Autodesk Inventor part; units mm, degrees
ref_plane "YZ Plane" through (0, 0, 0) normal (1, 0, 0) x (0, 1, 0)
ref_plane "XZ Plane" through (0, 0, 0) normal (0, 1, 0) x (-1, 0, 0)
ref_plane "XY Plane" through (0, 0, 0) normal (0, 0, 1) x (1, 0, 0)
sketch "Skizze1" plane through (0, 0, 0) normal (0, 1, 0) x (-1, 0, 0)
  line L0 (0, 0) -> (216, 0)
  line L1 (216, 0) -> (216, -42.3)
  line L2 (216, -42.3) -> (0, -42.3)
  line L3 (0, -42.3) -> (0, 0)
  dimension "d0" = 216
  dimension "d1" = 42.3
extrude "Extrusion1" add sketch "Skizze1" along normal blind 3
sketch "Skizze2" plane through (0, 6, 3) normal (0, 0, 1) x (1, 0, 0)
  line L0 (-216, 0) -> (0, 0)
  line L1 (0, 0) -> (0, 14)
  line L2 (0, 14) -> (-216, 14)
  line L3 (-216, 14) -> (-216, 0)
edge flange "Lasche1" height 20 angle 90 thickness 3 bend radius 3 thickness toward (0, 0, 1) relief tear relief width 3 relief depth 1.5 corner gap 3 corner form 0 edges at (-108, 3, 0) (-108, 3, -42.3) wall of the first edge with corners at (-216, 6, 3) (0, 6, 3) (0, 20, 3) (-216, 20, 3)
bend "Biegung1"
corner "Ecke1"
sketch "Skizze3" plane through (-218.1213, 3.8787, 0) normal (-0.7071068, -0.7071068, 0) x (0.7071068, -0.7071068, 0)
  line L0 (0, -42.3) -> (0, 0)
  line L1 (0, 0) -> (-17.5147, 0)
  line L2 (-17.5147, 0) -> (-17.5147, -42.3)
  line L3 (-17.5147, -42.3) -> (0, -42.3)
edge flange "Lasche2" height 20 angle 45 thickness 3 bend radius 3 thickness toward (-0.7071068, -0.7071068, 0) relief tear relief width 3 relief depth 1.5 corner gap 3 corner form 0 edges at (-216, 3, -21.15) (0, 3, -21.15) wall of the first edge with corners at (-218.1213, 3.8787, -42.3) (-218.1213, 3.8787, 0) (-230.5061, 16.2635, 0) (-230.5061, 16.2635, -42.3)
bend "Biegung2"
corner "Ecke2"
sketch "Skizze4" plane through (-216, 20, 6) normal (0, 0, 1) x (1, 0, 0)
  line L0 (0, 0) -> (0, -14)
  line L1 (0, -7) -> (216, -7)
  line L2 (216, 0) -> (216, -14)
  line L3 (0, 0) -> (216, 0)
  line L4 (108, 0) -> (108, -14)
  line L5 (216, -14) -> (0, -14)
  circle A0 centre (68, -7) radius 2.25
  circle A1 centre (18, -7) radius 2.25
  circle A2 centre (148, -7) radius 2.25
  circle A3 centre (198, -7) radius 2.25
  point P0 (216, -20)
  dimension "d25" = 4.5
  dimension "d26" = 4.5
  dimension "d27" = 4.5
  dimension "d28" = 4.5
  dimension "d29" = 80
  dimension "d30" = 180
extrude "Extrusion2" cut sketch "Skizze4" against normal blind 100 contours A1 L1 | L1 A1 | A0 L1 | L1 A0 | A2 L1 | L1 A2 | A3 L1 | L1 A3
fillet "Rundung1" radius 2 8 edges at (-231.5668, 15.2028, 0) (-231.5668, 15.2028, -42.3) (-216, 20, -46.8) (-216, 20, 4.5) (0, 20, 4.5) (15.5668, 15.2028, 0) (0, 20, -46.8) (15.5668, 15.2028, -42.3)
equation "\"d4\" = Stärke"
equation "\"d5\" = BreiteBiegungsfreistellung"
equation "\"d6\" = TiefeBiegungsfreistellung"
equation "\"d7\" = MinimalRest"
equation "\"d8\" = Übergangsradius"
equation "\"d11\" = Biegeradius"
equation "\"d12\" = GrößeEckenfreistellung"
equation "\"d13\" = Abstandsgröße"
equation "\"d14\" = JacobiRadiusGröße"
equation "\"d15\" = BreiteBiegungsfreistellung"
equation "\"d16\" = TiefeBiegungsfreistellung"
equation "\"d17\" = MinimalRest"
equation "\"d18\" = Übergangsradius"
equation "\"d21\" = Biegeradius"
equation "\"d22\" = GrößeEckenfreistellung"
equation "\"d23\" = Abstandsgröße"
equation "\"d24\" = JacobiRadiusGröße"
equation "\"Biegeradius\" = Stärke"
equation "\"BreiteBiegungsfreistellung\" = Stärke"
equation "\"TiefeBiegungsfreistellung\" = 0.5 * Stärke"
equation "\"GrößeEckenfreistellung\" = 4 * Stärke"
equation "\"MinimalRest\" = 2 * Stärke"
equation "\"Übergangsradius\" = Biegeradius"
equation "\"JacobiRadiusGröße\" = Biegeradius"
equation "\"Abstandsgröße\" = Stärke"
properties part number "Stossfänger_04" material "Aluminium 6061"
Could you check a few things on this model? Use its own coordinates, in mm. A direction names the side the tool comes from. Round coordinates to 2 decimals unless told otherwise and drop trailing zeros. Order: outer loops, then holes, each group sorted by start corner. A loop starts at its lowest first (then second) coordinate and runs counter-clockwise, first axis right, second up. Notation, with made-up numbers: M 41.25,-36.5 L 100.25,-36.5 A25 ccw 100.25,0.5 Z; hole C 27.25,26.25 d6. An arc over 180 degrees is marked long. One line per question, with ' | ' between items. Start each with the question number.
(1) For faces 5 (the face through (8, 7, -42.3)), 6 (the face through (8.227, 9.984, -21.446)), 7 (the face through (-106, 3, -21)), which set-ups out of +Z, -Z, +X, -X, +Y, -Y let a thin tool reach every point of the face, with its end or its side?
(2) Please list where these lines run through material, in increasing order: line 1 along X through (y, z) = (13, 4.55); line 2 along Z through (x, y) = (-153.5, 17.5); line 3 along Y through (x, z) = (-198, 5.2).
(3) Thinking about a two-plate mould opening in Y: for faces 1 (the face through (-226.522, 8.036, -20.854)), 2 (the face through (-16.79, 14.897, -46.779)), 3 (the face through (-195.854, 13.676, -46.779)), 4 (the face through (-216, 9, -46)), which applies, +Y half, -Y half, draft (parallel to the pull), parting line (faces both ways), or undercut?
(4) Suppose I cut it at A-A on x = -148. List the corners of the cut face in (y, z) for me, then the cut area to 3 significant figures.
(5) Suppose I cut it at B-B on z = -10.5. List the corners of the cut face in (x, y) for me, then the cut area to 3 significant figures.
(6) For P1, Ø3.5, axis at x = -18, y = 13, coming from the -Z side; P2, Ø1.5, axis at x = -204.5, z = -37.5, coming from the -Y side; P3, Ø3, axis at y = 5, z = -17.5, coming from the +X side; P4, Ø3, axis at y = 5.5, z = -26, coming from the +X side, each with a flat end and sliding along its axis, tell me the tip position at first contact or that it passes through.
Geometry results:
1) face 5: -Z, +X, +Y, -Y | face 6: +Z, -Z, +Y | face 7: +Y
2) line 1: -216 to -200.25, -195.75 to -150.25, -145.75 to -70.25, -65.75 to -20.25, -15.75 to 0 | line 2: -48.3 to -45.3, 3 to 6 | line 3: 3.01 to 10.75, 15.25 to 20
3) face 1: -Y half | face 2: undercut | face 3: undercut | face 4: draft
4) outline: M 0,-42.3 A6 ccw 6,-48.3 L 10.75,-48.3 L 10.75,-45.3 L 6,-45.3 A3 cw 3,-42.3 L 3,0 A3 cw 6,3 L 10.75,3 L 10.75,6 L 6,6 A6 ccw 0,0 Z; M 15.25,-48.3 L 20,-48.3 L 20,-45.3 L 15.25,-45.3 Z; M 15.25,3 L 20,3 L 20,6 L 15.25,6 Z | area: 226 mm²
5) outline: M -232.63,14.14 L -220.24,1.76 A6 ccw -216,0 L 0,0 A6 ccw 4.24,1.76 L 16.63,14.14 L 14.51,16.26 L 2.12,3.88 A3 cw 0,3 L -216,3 A3 cw -218.12,3.88 L -230.51,16.26 Z | area: 774 mm²
6) P1: through | P2: y = 0 | P3: x = 8.99 | P4: x = 9.49
